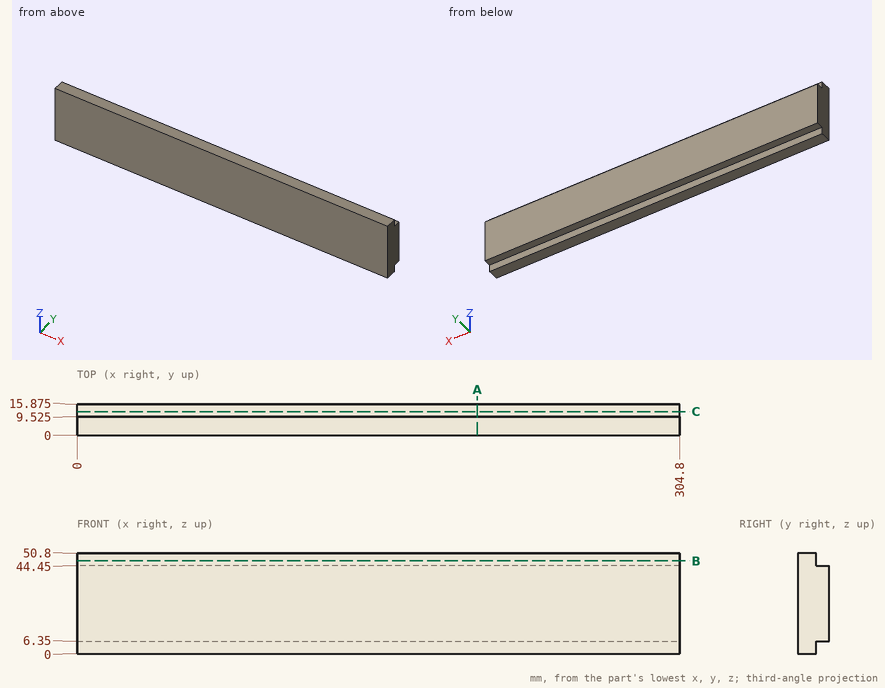
Source: three-view drawing plus pictorial views. Frame: mm from the lowest corner of the part. Coordinates: 2 decimals unless noted, no trailing zeros. Write each loop counter-clockwise with the first axis right and the second up, starting at its lowest first coordinate (ties: lowest second). Pieces come first, ordered by that corner, then holes. Notation, with made-up numbers: (5, 38) -> (40, 38) arc R22 ccw to (40, 54) -> close; hole circle Ø6 at (17.25, -4.75). An arc over 180 degrees is marked (long way). Answer as a JSON object with one key per item and string values.
1. Material intervals for line 1 (Z direction, x = 14, y = 11.5); line 2 (Y direction, x = 21.5, z = 44.5) (3 decimals), sorted ascending. Write a range as from..to.
Result set:
{"line 1": "z = 6.35..44.45", "line 2": "y = 0..9.525"}
2. First-contact query: P1, Ø8, axis at x = 116.5, y = 8, coming from the -Z side; P2, Ø1.9, axis at x = 163.5, z = 2.5, coming from the +Y side (3 decimals); P3, Ø1.9, axis at x = 119, y = 12, coming from the -Z side; P4, Ø5, axis at x = 180, y = 13.5, coming from the +Z side. Flat tips, straight axial feed; report the tip coordinate or a pass-through.
Result set:
{"P1": "stops at z = 0", "P2": "stops at y = 9.525", "P3": "stops at z = 6.35", "P4": "stops at z = 44.45"}
3. Section A-A on x = 202.5. Return the cut outline in (y, z) (3 decimals), then the cut area to 3 significant figures.
Result set:
{"outline": "(0, 0) -> (9.525, 0) -> (9.525, 6.35) -> (15.875, 6.35) -> (15.875, 44.45) -> (9.525, 44.45) -> (9.525, 50.8) -> (0, 50.8) -> close", "area": "726 mm2"}
4. Section B-B on z = 47. Return the cut outline in (x, y) (3 decimals).
Result set:
{"outline": "(0, 0) -> (304.8, 0) -> (304.8, 9.525) -> (0, 9.525) -> close"}
5. Section C-C on y = 12. Return the cut outline in (x, z), then the cut area to 3 significant figures.
Result set:
{"outline": "(0, 6.35) -> (304.8, 6.35) -> (304.8, 44.45) -> (0, 44.45) -> close", "area": "11,600 mm2"}
